Could you check a few things on this model? Use its own coordinates, in mm. Face numbers are marked on the shaded views. A direction names the side the tool comes from. Give positions to 0.01 mm unless a question says otherwise; leave off trailing zeros. Order: outer loops, then holes, each group sorted by start corner. A loop starts at its lowest first (then second) coordinate and runs counter-clockwise, first axis right, second up.
(1) Imagine slicing it at D-D, the plane x = -4.75. Write out the boundary of the cut face in (y, z).
(2) If we mould it in two halves opening along Z, with no side actions, what happens to the marked faces 1, 2 and 3? For each: released by +Z, released by -Z, zero draft, split by the parting line, or undercut.
(3) On a 3-axis mill with a long thin cutter (end or side, diameter ignored), from which of +Z, -Z, +X, -X, +Y, -Y can I reach the whole of each face in a straight line? I mean the marked faces 4, 5, 6 and 7. Say none if no direction works.
(4) Imagine slicing it at C-C, the plane y = 2. Write out the boundary of the cut face in (x, z), then the cut area to 3 significant figures.
(5) If I drill on probe 1 along Y at (x, z) = (3.5, 12.75); probe 2 along Z at (x, y) = (0, 3.2); probe 3 along Z at (x, y) = (1.25, 6.5), over which ranges is the centre line in solid material (lowest first)?
(6) Imagine slicing it at A-A, the plane x = 0. Write out the boundary of the cut face in (y, z), then the cut area to 3 significant figures.
(7) Imagine slicing it at B-B, the plane z = 6.5. Write out the boundary of the cut face in (x, y).
(8) Will these pins go through, and if not, where does the flat tip stop? pin 1 (1.7 mm diameter, centred on x = -3, y = -0.5, fed in from -Z); pin 2 (2 mm diameter, centred on x = -3.5, y = -2.5, fed in from -Z); pin 3 (5 mm diameter, centred on x = 3, y = 2.5, fed in from -Z).
from build123d import *

# Parameters (mm, degrees)
CYLINDER004_R        = 1.9
CYLINDER004_DEPTH    = 15
BOX005_W             = 15
BOX005_H             = 3.4
BOX005_DEPTH         = 17
ARRAY001_Y_COUNT     = 3
ARRAY001_Y_PITCH     = 6
CYLINDER003_R        = 7.5
CYLINDER003_DEPTH    = 15
BOX004_W             = 15
BOX004_H             = 15
BOX004_DEPTH         = 12.5
BODY_PLACEMENT_ANGLE = 180


with BuildPart() as side_2_bolt_hole:
    # Cylinder004 → Cylinder004 (new body)
    with BuildSketch(Plane(origin=(0, 7.5, 12.5), x_dir=(1, 0, 0), z_dir=(0, -1, 0))):
        Circle(CYLINDER004_R)
    extrude(amount=CYLINDER004_DEPTH)


with BuildPart() as side_2_extract_fusion:
    # Box005 → Box005 (new body)
    with BuildSketch(Plane(origin=(-7.5, -7.7, 3), x_dir=(1, 0, 0), z_dir=(0, 0, 1))):
        with Locations((7.5, 1.7)):
            Rectangle(BOX005_W, BOX005_H)
    extrude(amount=BOX005_DEPTH)

    # Array001 Y: side 2 extract fusion ×3


with BuildPart() as side_2_extract_fusion_1:
    add(side_2_extract_fusion.part)
    with Locations(*[(0, i * ARRAY001_Y_PITCH, 0) for i in range(1, ARRAY001_Y_COUNT)]):
        add(side_2_extract_fusion.part)

    # Fusion004: union side 2 bolt hole
    add(side_2_bolt_hole.part)


with BuildPart() as outer_cylinder001:
    # Cylinder003 → Cylinder003 (new body)
    with BuildSketch(Plane(origin=(0, 7.5, 12.5), x_dir=(1, 0, 0), z_dir=(0, -1, 0))):
        Circle(CYLINDER003_R)
    extrude(amount=CYLINDER003_DEPTH)


with BuildPart() as side_2_cut_clone:
    # Box004 → Box004 (new body)
    with BuildSketch(Plane(origin=(-7.5, -7.5, 0), x_dir=(1, 0, 0), z_dir=(0, 0, 1))):
        with Locations((7.5, 7.5)):
            Rectangle(BOX004_W, BOX004_H)
    extrude(amount=BOX004_DEPTH)

    # Fusion003: union outer cylinder001
    add(outer_cylinder001.part)

    # Cut001: cut side 2 extract fusion
    add(side_2_extract_fusion_1.part, mode=Mode.SUBTRACT)


with BuildPart() as side_2_cut_clone_1:
    # Body placement: moved
    add(side_2_cut_clone.part.moved(Location((0, 0, 25))).rotate(Axis((0, 0, 25), (0, 1, 0)), BODY_PLACEMENT_ANGLE))


solid = side_2_cut_clone_1.part
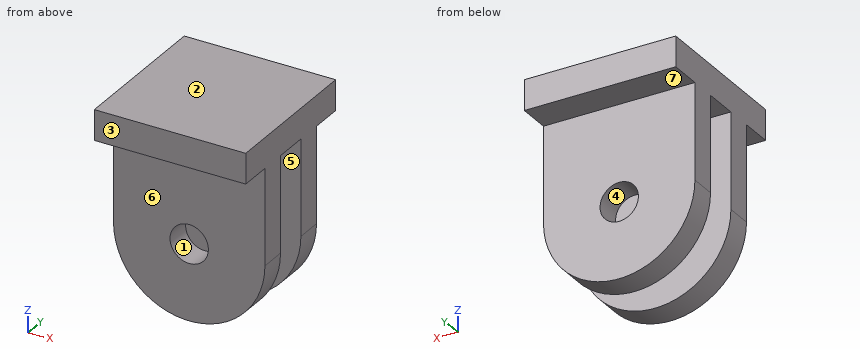
Answer block:
1. outline: (-7.5, 22) - (-4.3, 22) - (-4.3, 6.7) - (-1.7, 6.7) - (-1.7, 22) - (1.7, 22) - (1.7, 6.7) - (4.3, 6.7) - (4.3, 22) - (7.5, 22) - (7.5, 25) - (-7.5, 25) - close
2. face 1: undercut
2. face 2: released by +Z
2. face 3: zero draft
3. face 4: +Y, -Y
3. face 5: -Z, +X, -X
3. face 6: -Z, +X, -X, -Y
3. face 7: -Z, +X, -X, +Y
4. outline: (-7.5, 12.5) arc R7.5 ccw to (7.5, 12.5) - (7.5, 25) - (-7.5, 25) - close; hole circle Ø3.8 at (0, 12.5)
4. area: 265 mm2
5. probe 1: y = -4.3 to -1.7, 1.7 to 4.3
5. probe 2: z = 5 to 10.6, 14.4 to 25
5. probe 3: z = 22 to 25
6. outline: (-7.5, 22) - (-4.3, 22) - (-4.3, 14.4) - (-1.7, 14.4) - (-1.7, 22) - (1.7, 22) - (1.7, 14.4) - (4.3, 14.4) - (4.3, 22) - (7.5, 22) - (7.5, 25) - (-7.5, 25) - close; (-4.3, 5) - (-1.7, 5) - (-1.7, 10.6) - (-4.3, 10.6) - close; (1.7, 5) - (4.3, 5) - (4.3, 10.6) - (1.7, 10.6) - close
6. area: 114 mm2
7. outline: (-4.5, -4.3) - (4.5, -4.3) - (4.5, -1.7) - (-4.5, -1.7) - close; (-4.5, 1.7) - (4.5, 1.7) - (4.5, 4.3) - (-4.5, 4.3) - close
8. pin 1: stops at z = 22
8. pin 2: stops at z = 5.43
8. pin 3: stops at z = 5.02
